```python
from build123d import *

# Parameters (mm, degrees)
F0_R     = 44.45
F1_DEPTH = 19.05
F2_R     = 6.35
F2_R_2   = 6.191887
F2_R_3   = 5.749023
F3_DEPTH = 25.4
F4_R     = 9.525
F4_R_2   = 4.796192
F5_DEPTH = 6.35


with BuildPart() as f1:
    # F0 (on Front) → F1 (new body)
    with BuildSketch(Plane.XZ):
        Circle(F0_R)
    extrude(amount=F1_DEPTH)

    # F2 (on face) → F3 (cut)
    with BuildSketch(Plane.XZ.offset(19.05)):
        with Locations((0, 25.000811)):
            Circle(F2_R)
        with Locations((0, -25.407325)):
            Circle(F2_R)
        with Locations((26.017097, 0)):
            Circle(F2_R)
        with Locations((-26.830139, 0)):
            Circle(F2_R)
        with Locations((18.185616, 17.9583)):
            Circle(F2_R_2)
        with Locations((19.16673, -17.569499)):
            Circle(F2_R_3)
        with Locations((-17.886758, -18.090015)):
            Circle(F2_R)
        with Locations((-19.512825, 18.496535)):
            Circle(F2_R)
    extrude(amount=-F3_DEPTH, mode=Mode.SUBTRACT)

    # F4 (on face) → F5 (join)
    with BuildSketch(Plane.XZ.offset(19.05)):
        Circle(F4_R)
        Circle(F4_R_2, mode=Mode.SUBTRACT)
    extrude(amount=F5_DEPTH)


solid = f1.part
```
Part model, mm, in its own coordinate system. A direction names the side the tool comes from. Coordinates: 2 decimals unless noted, no trailing zeros. Order: outer loops, then holes, each group sorted by start corner. A loop starts at its lowest first (then second) coordinate and runs counter-clockwise, first axis right, second up. Notation, with made-up numbers: (61, -6.75) - (116, -6.75) arc R25 cw to (116, 26.25) - close; hole circle Ø6 at (-38.75, -6.5). An arc over 180 degrees is marked (long way). Return JSON: item names as keys, results as strings. Group by question number.
Item 1: Cut at D-D (x = -22). List the corners of the cut face in (y, z).
Item 2: Pin check, flat tips, straight feed: pin 1 (5 mm diameter, centred on y = -16, z = -14, fed in from -X); pin 2 (5 mm diameter, centred on x = 28.5, y = -14.5, fed in from +Z); pin 3 (1 mm diameter, centred on x = -27.5, z = 4, fed in from +Y); pin 4 (2 mm diameter, centred on x = 17.5, y = -12.5, fed in from +Z). Stop position of each tip, or through.
Item 3: Cut at A-A (x = 0). List the corners of the cut face in (y, z) (3 decimals).
Item 4: Pull direction X, two halves, no side cores. Call faces 3 (the face through (-4.4, -25.4, 2.3)), 4 (the face through (42.397, -9.392, 13.352)), 5 (the face through (13.62, -9.66, 22.14)): pulls with the +X half, pulls with the -X half, needs draft (parallel to the pull), parting line crosses it, or undercut.
Item 5: Drill centre lines: probe 1 along Z at (x, y) = (0, -8.75); probe 2 along X at (y, z) = (-6.25, -21); probe 3 along X at (y, z) = (-9.25, -18.5). Where is each one in solid material? Low to high. Write a range as from..to.
Item 6: Which spindle directions (+Z, -Z, +X, -X, +Y, -Y) get a long thin tool onto all of the face, cutting with end or side? Do faces 1 (the face through (-33.174, -9.658, 0.279)), 2 (the face through (-7.559, -22.181, -5.796)). Say none if no direction does.
Item 7: Cut at B-B (z = 0). List the corners of the cut face in (x, y) (3 decimals), plus the area to 3 significant figures.
Item 8: Cut at C-C (y = -20.75). List the corners of the cut face in (x, z) (3 decimals).
Check values:
{
 "1": {"outline": "(-19.05, -38.62) - (0, -38.62) - (0, -22.93) - (-19.05, -22.93) - close; (-19.05, -13.25) - (0, -13.25) - (0, -4.12) - (-19.05, -4.12) - close; (-19.05, 4.12) - (0, 4.12) - (0, 12.65) - (-19.05, 12.65) - close; (-19.05, 24.34) - (0, 24.34) - (0, 38.62) - (-19.05, 38.62) - close"},
 "2": {"pin 1": "stops at x = -42.94", "pin 2": "stops at z = 36.05", "pin 3": "passes through", "pin 4": "stops at z = 41.27"},
 "3": {"outline": "(-25.4, -9.525) - (-19.05, -9.525) - (-19.05, -19.057) - (0, -19.057) - (0, 18.651) - (-19.05, 18.651) - (-19.05, 9.525) - (-25.4, 9.525) - (-25.4, 4.796) - (-19.05, 4.796) - (-19.05, -4.796) - (-25.4, -4.796) - close; (-19.05, -44.45) - (0, -44.45) - (0, -31.757) - (-19.05, -31.757) - close; (-19.05, 31.351) - (0, 31.351) - (0, 44.45) - (-19.05, 44.45) - close"},
 "4": {"face 3": "needs draft", "face 4": "parting line crosses it", "face 5": "undercut"},
 "5": {"probe 1": "z = -44.45..-31.76, -19.06..18.65, 31.35..44.45", "probe 2": "x = -39.18..-23.53, -12.24..-4.57, 4.57..14.55, 23.78..39.18", "probe 3": "x = -40.42..-24.22, -11.55..13.49, 24.84..40.42"},
 "6": {"face 1": "+Y, -Y", "face 2": "-Y"},
 "7": {"outline": "(-44.45, -19.05) - (-33.18, -19.05) - (-33.18, 0) - (-44.45, 0) - close; (-20.48, -19.05) - (-9.525, -19.05) - (-9.525, -25.4) - (-4.796, -25.4) - (-4.796, -19.05) - (4.796, -19.05) - (4.796, -25.4) - (9.525, -25.4) - (9.525, -19.05) - (19.667, -19.05) - (19.667, 0) - (-20.48, 0) - close; (32.367, -19.05) - (44.45, -19.05) - (44.45, 0) - (32.367, 0) - close", "area": "1,270 mm2"},
 "8": {"outline": "circle Ø19.05 at (0, 0); hole circle Ø9.592 at (0, 0)"}
}
